Work out the finished part from the listing and answer in its coordinate system (mm). A direction names the side the tool comes from. Round coordinates to 2 decimals unless told otherwise and drop trailing zeros. Write each loop counter-clockwise with the first axis right and the second up, starting at its lowest first coordinate (ties: lowest second). Pieces come first, ordered by that corner, then holes.
from build123d import *

# Parameters (mm, degrees)
SKETCH060_R     = 1.5
PAD035_DEPTH    = 4
SKETCH061_R     = 2.5
POCKET025_DEPTH = 2
SKETCH048_W     = 5
SKETCH048_H     = 4
POCKET019_DEPTH = 5
FILLET012_R     = 2
FILLET013_R     = 2
SKETCH049_R     = 4
POCKET020_DEPTH = 4


with BuildPart() as part:
    # Sketch060 (on CopyDatumPlane) → Pad035 (new body)
    with BuildSketch(Plane(origin=(0, 20, 0), x_dir=(1, 0, 0), z_dir=(0, 1, 0))):
        Polygon((-30, 28), (30, 28), (30, 15.2), (26.8, 15.2), (26.8, -15), (-26.8, -15), (-26.8, 15.2), (-30, 15.2), align=None)
        with Locations((-22.5, 25)):
            Circle(SKETCH060_R, mode=Mode.SUBTRACT)
        with Locations((22.5, 25)):
            Circle(SKETCH060_R, mode=Mode.SUBTRACT)
        with Locations((22.5, -12)):
            Circle(SKETCH060_R, mode=Mode.SUBTRACT)
        with Locations((-22.5, -12)):
            Circle(SKETCH060_R, mode=Mode.SUBTRACT)
    extrude(amount=PAD035_DEPTH)

    # Sketch061 (on Face14 of Pad035) → Pocket025 (cut)
    with BuildSketch(Plane(origin=(0, 24, 0), x_dir=(1, 0, 0), z_dir=(0, 1, 0))):
        with Locations((-22.5, 25)):
            Circle(SKETCH061_R)
        with Locations((22.5, 25)):
            Circle(SKETCH061_R)
        with Locations((22.5, -12)):
            Circle(SKETCH061_R)
        with Locations((-22.5, -12)):
            Circle(SKETCH061_R)
    extrude(amount=-POCKET025_DEPTH, mode=Mode.SUBTRACT)

    # Sketch048 (on Face1 of Pocket025) → Pocket019 (cut)
    with BuildSketch(Plane(origin=(0, 20, -28), x_dir=(-1, 0, 0), z_dir=(0, 0, -1))):
        with Locations((-17, 2)):
            Rectangle(SKETCH048_W, SKETCH048_H)
    extrude(amount=-POCKET019_DEPTH, mode=Mode.SUBTRACT)

    # Fillet012
    fillet012_edges = [part.edges().sort_by_distance(p)[0] for p in [
        (19.5, 22, -23),
    ]]
    fillet(fillet012_edges, radius=FILLET012_R)

    # Fillet013
    fillet013_edges = [part.edges().sort_by_distance(p)[0] for p in [
        (14.5, 22, -23),
    ]]
    fillet(fillet013_edges, radius=FILLET013_R)

    # Sketch049 (on Face20 of Fillet013) → Pocket020 (cut)
    with BuildSketch(Plane(origin=(0, 24, 0), x_dir=(1, 0, 0), z_dir=(0, 1, 0))):
        with Locations((10, -8)):
            Circle(SKETCH049_R)
    extrude(amount=-POCKET020_DEPTH, mode=Mode.SUBTRACT)


solid = part.part
Q1. Find the intervals of material crossed by L1, parallel to Z at x = 22.5, y = 20.55; L2, parallel to Z at x = 22.5, y = 22.4; L3, parallel to X at y = 22.7, z = 8.5, in increasing order.
Q2. A tool of negligible diameter and unlimited length cuts with its end or side. For faces 1 (the face through (-24, 21, 12)), 2 (the face through (28, 22, -15.2)), 3 (the face through (-24, 23, -27)), 4 (the face through (18.93, 22.03, -23.6)), from which of +Z, -Z, +X, -X, +Y, -Y can it reach the whole face along a straight path? Write none if from no direction.
Q3. The mould has two halves that part along Z. Classify faces 5 (the face through (30, 22, -22)), 6 (the face through (-24, 23, 14)), 7 (the face through (0, 22, 15)): +Z half, -Z half, draft (parallel to the pull), parting line (faces both ways), or undercut.
Q4. Find section A-A (y = 23.15). Determine the outline of the cut face in (x, z), plus the area to 3 significant figures.
Q5. Find section D-D (z = -13.5). Determine the outline of the cut face in (x, y), plus the area to 3 significant figures.
Q6. Given pin 1 (3.5 mm diameter, centred on x = 22.5, z = -25, fed in from +Y); pin 2 (1.6 mm diameter, centred on x = -28, y = 22, fed in from +Z); pin 3 (1.5 mm diameter, centred on x = 23, z = 12, fed in from +Y); pin 4 (1.1 mm diameter, centred on x = 17, y = 23, fed in from -Z), each flat-ended and moving along its own axis, determine where each tip first touches the part or whether it passes through.
Q7. Find section B-B (x = 22.5). Determine the outline of the cut face in (y, z), plus the area to 3 significant figures.
Q8. Find section C-C (x = 11). Determine the outline of the cut face in (y, z), plus the area to 3 significant figures.
Report:
1. L1: z = -28 to -26.5, -23.5 to 10.5, 13.5 to 15
1. L2: z = -28 to -27.5, -22.5 to 9.5, 14.5 to 15
1. L3: x = -26.8 to 6.03, 13.97 to 26.8
2. face 1: +Y, -Y
2. face 2: +Z, +X, +Y, -Y
2. face 3: +Y
2. face 4: -Z, +Y, -Y
3. face 5: draft
3. face 6: undercut
3. face 7: +Z half
4. outline: (-30, -28) - (14.5, -28) - (14.5, -25) arc R2 cw to (16.5, -23) - (17.5, -23) arc R2 cw to (19.5, -25) - (19.5, -28) - (30, -28) - (30, -15.2) - (26.8, -15.2) - (26.8, 15) - (-26.8, 15) - (-26.8, -15.2) - (-30, -15.2) - close; hole circle Ø5 at (-22.5, -25); hole circle Ø5 at (-22.5, 12); hole circle Ø8 at (10, 8); hole circle Ø5 at (22.5, -25); hole circle Ø5 at (22.5, 12)
4. area: 2,230 mm2
5. outline: (-26.8, 20) - (26.8, 20) - (26.8, 24) - (-26.8, 24) - close
5. area: 214 mm2
6. pin 1: stops at y = 22
6. pin 2: stops at z = -15.2
6. pin 3: passes through
6. pin 4: stops at z = -23
7. outline: (20, -28) - (24, -28) - (24, -27.5) - (22, -27.5) - (22, -26.5) - (20, -26.5) - close; (20, -23.5) - (22, -23.5) - (22, -22.5) - (24, -22.5) - (24, 9.5) - (22, 9.5) - (22, 10.5) - (20, 10.5) - close; (20, 13.5) - (22, 13.5) - (22, 14.5) - (24, 14.5) - (24, 15) - (20, 15) - close
7. area: 140 mm2
8. outline: (20, -28) - (24, -28) - (24, 4.13) - (20, 4.13) - close; (20, 11.87) - (24, 11.87) - (24, 15) - (20, 15) - close
8. area: 141 mm2
